Source: CAD feature listing. Evaluate the final solid. Frame: model axes, mm. Face numbers are marked on the shaded views. Give positions to 0.01 mm unless a question says otherwise; leave off trailing zeros. Order: outer loops, then holes, each group sorted by start corner. A loop starts at its lowest first (then second) coordinate and runs counter-clockwise, first axis right, second up. Notation, with made-up numbers: M 86,19 L 115,19 A23 ccw 115,55 Z; hole C 86.5,35 d7. An arc over 180 degrees is marked long. Use CSV: the item, a comma, the result in double quotes. Start each with the question number.
1. Line query: line 1 along X through (y, z) = (9.75, 7.62); line 2 along X through (y, z) = (-5, 7.62); line 3 along X through (y, z) = (-6, 7.62). Output: solid intervals per line, ascending. Write a range as [from, to].
2. Mould query, pull axis X, two halves, no side actions, for the marked faces 1, 2 and 3. Classes: released by +X, released by -X, zero draft, split by the parting line, or undercut.
3. Section query C-C, the plane x = 0. Return the cut outline in (y, z).
4. Section query B-B, the plane y = 0. Return the cut outline in (x, z), plus the area to 3 significant figures.
5. Section query D-D, the plane y = -4.75. Return the cut outline in (x, z) (1 decimal).
6. Pin query (flat end, axial travel): P1, Ø4, axis at x = 4, y = 3, coming from the +Z side; P2, Ø1.9, axis at x = 7.62, z = 7.62, coming from the +Y side. Return the tip coordinate at first contact, or that it passes through.
7. Section query A-A, the plane z = 15. Return the cut outline in (x, y) (3 decimals).
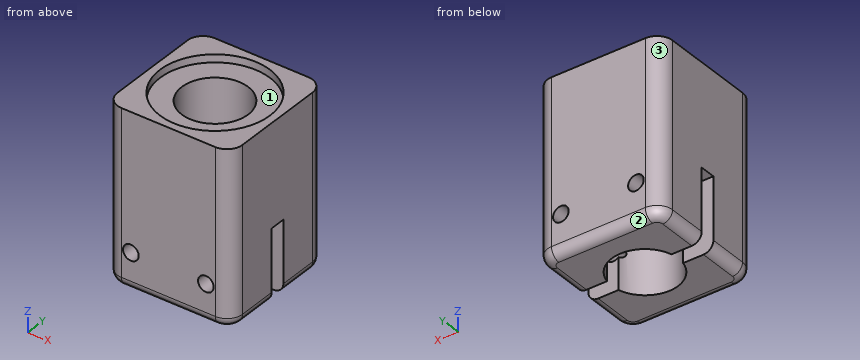
from build123d import *

# Parameters (mm, degrees)
F1_DEPTH  = 36.093
F3_D      = 13.49248
F4_R      = 11.176
F5_DEPTH  = 1.5875
F7_DEPTH  = 25.401
F8_R      = 1.5875
F9_DEPTH  = 25.401
F10_R     = 2
F11_DEPTH = 0.845
F12_DEPTH = 0.845
F13_DEPTH = 0.889


with BuildPart() as f1:
    # F0 (on Top) → F1 (new body)
    with BuildSketch(Plane.XY):
        with BuildLine():
            Line((9.525, 12.7), (-9.525, 12.7))
            ThreePointArc((-9.525, 12.7), (-11.7700640303, 11.7700640303), (-12.7, 9.525))
            Line((-12.7, 9.525), (-12.7, -9.525))
            ThreePointArc((-12.7, -9.525), (-11.7700640303, -11.7700640303), (-9.525, -12.7))
            Line((-9.525, -12.7), (9.525, -12.7))
            ThreePointArc((9.525, -12.7), (11.7700640303, -11.7700640303), (12.7, -9.525))
            Line((12.7, -9.525), (12.7, 9.525))
            ThreePointArc((12.7, 9.525), (11.7700640303, 11.7700640303), (9.525, 12.7))
        make_face()
    extrude(amount=F1_DEPTH)

    # F3 (through all)
    with Locations(Plane.XY.offset(36.093)):
        with Locations((0, 0)):
            Hole(F3_D / 2)

    # F4 (on face) → F5 (cut)
    with BuildSketch(Plane.XY.offset(36.093)):
        Circle(F4_R)
    extrude(amount=-F5_DEPTH, mode=Mode.SUBTRACT)

    # F6 (on face) → F7 (cut, through all)
    with BuildSketch(Plane(origin=(-12.7, 0, 0), x_dir=(0, -1, 0), z_dir=(-1, 0, 0))):
        Polygon((1.5875, 15.4555), (0, 15.4555), (-1.5875, 15.4555), (-1.5875, -0.7945992402), (1.5875, -1.3757834677), align=None)
    extrude(amount=-F7_DEPTH, mode=Mode.SUBTRACT)

    # F8 (on face) → F9 (cut, through all)
    with BuildSketch(Plane.XZ.offset(12.7)):
        with Locations((-7.62, 7.62)):
            Circle(F8_R)
        with Locations((7.62, 7.62)):
            Circle(F8_R)
    extrude(amount=-F9_DEPTH, mode=Mode.SUBTRACT)

    # F10
    f10_edges = [f1.edges().sort_by_distance(p)[0] for p in [
        (-12.7, 5.55625, 0),
        (-12.7, -5.55625, 0),
    ]]
    fillet(f10_edges, radius=F10_R)

    # F11 (cut): a face of the model
    f11_faces = [f1.faces().sort_by_distance(p)[0] for p in [
        (0, 12.3407897552, 36.093),
    ]]
    extrude(f11_faces, amount=-F11_DEPTH, mode=Mode.SUBTRACT)

    # F12 (cut): a face of the model
    f12_faces = [f1.faces().sort_by_distance(p)[0] for p in [
        (-10.8598949845, 0, 34.5055),
    ]]
    extrude(f12_faces, amount=-F12_DEPTH, mode=Mode.SUBTRACT)

    # F13 (add): faces of the model
    f13_faces = [f1.faces().sort_by_distance(p)[0] for p in [
        (9.6914617735, 0, 15.4555),
        (-9.6914617735, 0, 15.4555),
    ]]
    extrude(f13_faces, amount=F13_DEPTH)


solid = f1.part
Result set:
1,line 1,"[-12.69, -9.21], [-6.03, 6.03], [9.21, 12.69]"
1,line 2,"[-12.7, -9.21], [-6.03, -4.53], [4.53, 6.03], [9.21, 12.7]"
1,line 3,"[-12.7, -9.21], [-6.03, -3.08], [3.08, 6.03], [9.21, 12.7]"
2,face 1,"undercut"
2,face 2,"zero draft"
2,face 3,"released by -X"
3,outline,"M -12.7,2 A2 ccw -10.7,0 L -6.75,0 L -6.75,33.66 L -11.18,33.66 L -11.18,35.25 L -12.7,35.25 Z; M 6.75,0 L 10.7,0 A2 ccw 12.7,2 L 12.7,35.25 L 11.18,35.25 L 11.18,33.66 L 6.75,33.66 Z"
4,outline,"M -12.7,14.57 L -6.75,14.57 L -6.75,33.66 L -11.18,33.66 L -11.18,35.25 L -12.7,35.25 Z; M 6.75,14.57 L 12.7,14.57 L 12.7,35.25 L 11.18,35.25 L 11.18,33.66 L 6.75,33.66 Z"
4,area,"232 mm2"
5,outline,"M -12.7,2 A2 ccw -10.7,0 L -4.8,0 L -4.8,33.7 L -10.1,33.7 L -10.1,35.2 L -12.7,35.2 Z; M 4.8,0 L 10.7,0 A2 ccw 12.7,2 L 12.7,35.2 L 10.1,35.2 L 10.1,33.7 L 4.8,33.7 Z; hole C -7.6,7.6 d3.2; hole C 7.6,7.6 d3.2"
6,P1,"z = 33.66"
6,P2,"through"
7,outline,"M -12.7,-9.525 A3.175 ccw -9.525,-12.7 L 9.525,-12.7 A3.175 ccw 12.7,-9.525 L 12.7,9.525 A3.175 ccw 9.525,12.7 L -9.525,12.7 A3.175 ccw -12.7,9.525 Z; hole C 0,0 d13.492"
